from build123d import *

# Parameters (mm, degrees)
SKETCH2_W           = 40
SKETCH2_H           = 40
BOSS_EXTRUDE1_DEPTH = 5
SKETCH3_W           = 40
SKETCH3_H           = 5
BOSS_EXTRUDE2_DEPTH = 10
SKETCH4_W           = 5
SKETCH4_H           = 40
BOSS_EXTRUDE3_DEPTH = 80


with BuildPart() as part:
    # Sketch2 → Boss-Extrude1 (new body)
    with BuildSketch(Plane(origin=(0, 0, 0), x_dir=(1, 0, 0), z_dir=(0, 1, 0))):
        Rectangle(SKETCH2_W, SKETCH2_H)
    extrude(amount=BOSS_EXTRUDE1_DEPTH)

    # Sketch3 → Boss-Extrude2 (add)
    with BuildSketch(Plane(origin=(20, 0, 0), x_dir=(0, 0, -1), z_dir=(1, 0, 0))):
        with Locations((0, 2.5)):
            Rectangle(SKETCH3_W, SKETCH3_H)
    extrude(amount=BOSS_EXTRUDE2_DEPTH)

    # Sketch4 → Boss-Extrude3 (add)
    with BuildSketch(Plane(origin=(0, 5, 0), x_dir=(1, 0, 0), z_dir=(0, 1, 0))):
        with Locations((-17.5, 0)):
            Rectangle(SKETCH4_W, SKETCH4_H)
        with Locations((27.5, 0)):
            Rectangle(SKETCH4_W, SKETCH4_H)
    extrude(amount=BOSS_EXTRUDE3_DEPTH)


solid = part.part
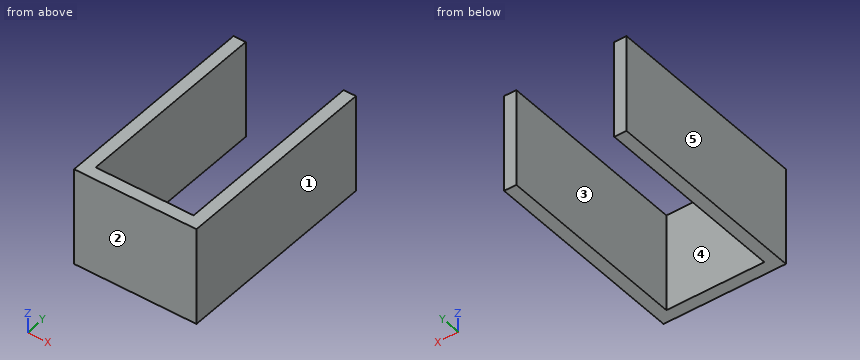
Could you check a few things on this model? Use its own coordinates, in mm. Face numbers are marked on the shaded views. A direction names the side the tool comes from. Give positions to 0.01 mm unless a question says otherwise; leave off trailing zeros. Loops run counter-clockwise (first coordinate to the right, second up) from the corner with the lowest first, then second, coordinate; pieces in that order, holes last. Notation, with made-up numbers: M 80.5,56.25 L 139.5,56.25 A20 cw 139.5,64.25 Z; hole C 32,-22 d4. An arc over 180 degrees is marked long. Answer as a JSON object with one key per item and string values.
Q1. Suppose I cut it at A-A, the plane y = 50. List the corners of the cut face in (x, z) for me.
Values found:
{"outline": "M -20,-20 L -15,-20 L -15,20 L -20,20 Z; M 25,-20 L 30,-20 L 30,20 L 25,20 Z"}
Q2. For the marked faces 4 and 5, which set-ups out of +Z, -Z, +X, -X, +Y, -Y let a thin tool reach every point of the face, with its end or its side?
Values found:
{"face 4": "+Z, -Z, +Y", "face 5": "+Z, -Z, -X, +Y, -Y"}
Q3. If I drill on probe 1 along X at (y, z) = (24.5, -5); probe 2 along Y at (x, z) = (-8.5, -17), over which ranges is the centre line in solid material (lowest first)? Write a range as [from, to].
Values found:
{"probe 1": "x = [-20, -15], [25, 30]", "probe 2": "y = [0, 5]"}
Q4. Suppose I cut it at B-B, the plane z = -9. List the corners of the cut face in (x, y) for me.
Values found:
{"outline": "M -20,0 L 30,0 L 30,85 L 25,85 L 25,5 L -15,5 L -15,85 L -20,85 Z"}
Q5. For P1, Ø1, axis at x = 4, z = -8.5, coming from the -Y side; P2, Ø20, axis at x = 7.5, z = -9.5, coming from the +Y side, each with a flat end and sliding along its axis, tell me the tip position at first contact or that it passes through.
Values found:
{"P1": "stops at y = 0", "P2": "stops at y = 5"}
Q6. Suppose I cut it at C-C, the plane x = 22.5. List the corners of the cut face in (y, z) for me, plus the area to 3 significant figures.
Values found:
{"outline": "M 0,-20 L 5,-20 L 5,20 L 0,20 Z", "area": "200 mm²"}
Q7. If we mould it in two halves opening along X, with no side actions, what happens to the marked faces 1, 2 and 3? For each: pulls with the +X half, pulls with the -X half, needs draft (parallel to the pull), parting line crosses it, or undercut.
Values found:
{"face 1": "pulls with the +X half", "face 2": "needs draft", "face 3": "undercut"}
